The drawing under review shows one solid part. Ordinate dimensions are in mm from its lowest x, y, z. Coordinates: 2 decimals unless noted, no trailing zeros. Write each loop counter-clockwise with the first axis right and the second up, starting at its lowest first coordinate (ties: lowest second). Pieces come first, ordered by that corner, then holes. Notation, with made-up numbers: M -19,11 L 31,11 A14 ccw 31,23 Z; hole C 3.25,79.25 d2. An arc over 180 degrees is marked long. Write item = value, one per line.
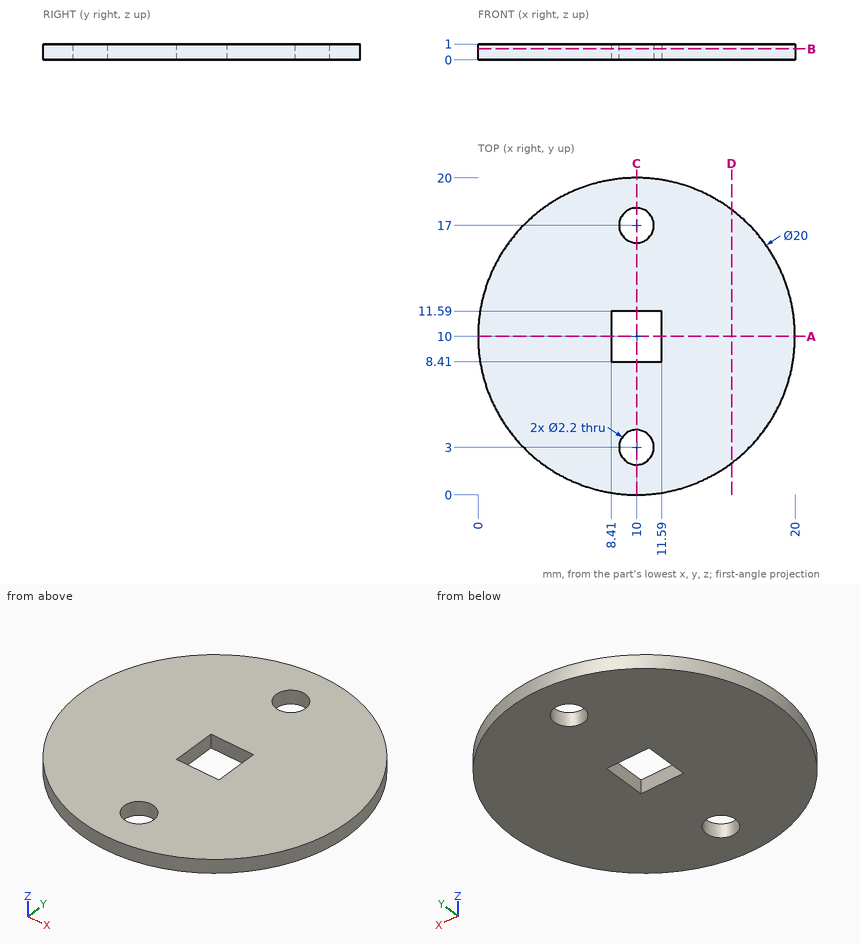
Q1. Consider section B-B, the plane z = 0.7. State the section outline as (x, y) points, and give its area (3 significant figures).
Check result:
outline = C 10,10 d20; hole M 8.41,8.41 L 11.59,8.41 L 11.59,11.59 L 8.41,11.59 Z; hole C 10,3 d2.2; hole C 10,17 d2.2
area = 296 mm²
Q2. Wall thickness on line 1 (Y direction, x = 10, z = 0.4); line 2 (Y direction, x = 9.25, z = 0.75); line 3 (X direction, y = 9.5, z = 0.1): over which ranges is each line inside the solid? List them lowest first.
Check result:
line_1 = 0 to 1.9, 4.1 to 8.41, 11.59 to 15.9, 18.1 to 20
line_2 = 0.03 to 2.2, 3.8 to 8.41, 11.59 to 16.2, 17.8 to 19.97
line_3 = 0.01 to 8.41, 11.59 to 19.99
Q3. Consider section A-A, the plane y = 10. State the section outline as (x, z) points.
Check result:
outline = M 0,0 L 8.41,0 L 8.41,1 L 0,1 Z; M 11.59,0 L 20,0 L 20,1 L 11.59,1 Z
Q4. Consider section D-D, the plane x = 16. State the section outline as (y, z) points, and give its area (3 significant figures).
Check result:
outline = M 2,0 L 18,0 L 18,1 L 2,1 Z
area = 16.0 mm²
Q5. For P1, Ø1.8, axis at x = 10, y = 17, coming from the +Z side (3 decimals), flat-tipped, find the tip position at first contact; note if it passes through.
Check result:
P1 = through
Q6. Consider section C-C, the plane x = 10. State the section outline as (y, z) points, and give its area (3 significant figures).
Check result:
outline = M 0,0 L 1.9,0 L 1.9,1 L 0,1 Z; M 4.1,0 L 8.41,0 L 8.41,1 L 4.1,1 Z; M 11.59,0 L 15.9,0 L 15.9,1 L 11.59,1 Z; M 18.1,0 L 20,0 L 20,1 L 18.1,1 Z
area = 12.4 mm²
